Work out the finished part from the listing and answer in its coordinate system (mm). A direction names the side the tool comes from. Coordinates: 2 decimals unless noted, no trailing zeros. Order: outer loops, then holes, each group sorted by start corner. A loop starts at its lowest first (then second) coordinate and runs counter-clockwise, first axis right, second up. Notation, with made-up numbers: (36.25, 0) - (77.25, 0) arc R30 ccw to (77.25, 32) - close; hole circle Ø11 at (40.25, -6.75). An arc over 180 degrees is marked (long way). Use CSV: the item, a comma, the result in double quotes. Start each with the question number.
Autodesk Inventor part; units mm, degrees
ref_plane "YZ Plane" through (0, 0, 0) normal (1, 0, 0) x (0, 1, 0)
ref_plane "XZ Plane" through (0, 0, 0) normal (0, 1, 0) x (-1, 0, 0)
ref_plane "XY Plane" through (0, 0, 0) normal (0, 0, 1) x (1, 0, 0)
sketch "Sketch1" plane through (0, 0, 0) normal (0, 0, 1) x (1, 0, 0)
  line L0 (-105.7, 0) -> (105.7, 0) construction
  line L1 (0, -31.15) -> (0, 31.15) construction
  line L2 (-75.5, 22.25) -> (75.5, 22.25)
  line L3 (75.5, 22.25) -> (75.5, -22.25)
  line L4 (75.5, -22.25) -> (-75.5, -22.25)
  line L5 (-75.5, -22.25) -> (-75.5, 22.25)
  line L6 (-49.21, 1.55) -> (-49.21, -1.55) construction
  line L7 (-56.21, 1.55) -> (-56.21, -1.55)
  line L8 (-42.21, -1.55) -> (-42.21, 1.55)
  arc A0 (-42.21, 1.55) -> (-56.21, 1.55) centre (-49.21, 1.55) ccw
  arc A1 (-56.21, -1.55) -> (-42.21, -1.55) centre (-49.21, -1.55) ccw
  line L9 (49.21, 1.55) -> (49.21, -1.55) construction
  line L10 (56.21, 1.55) -> (56.21, -1.55)
  line L11 (42.21, -1.55) -> (42.21, 1.55)
  arc A2 (56.21, 1.55) -> (42.21, 1.55) centre (49.21, 1.55) ccw
  arc A3 (42.21, -1.55) -> (56.21, -1.55) centre (49.21, -1.55) ccw
  line L12 (-49.21, 1.55) -> (-49.21, -1.55) construction
  line L13 (-59.71, 1.55) -> (-59.71, -1.55)
  line L14 (-38.71, -1.55) -> (-38.71, 1.55)
  arc A4 (-38.71, 1.55) -> (-59.71, 1.55) centre (-49.21, 1.55) ccw
  arc A5 (-59.71, -1.55) -> (-38.71, -1.55) centre (-49.21, -1.55) ccw
  line L15 (59.71, 1.55) -> (59.71, -1.55)
  line L16 (38.71, -1.55) -> (38.71, 1.55)
  arc A6 (59.71, 1.55) -> (38.71, 1.55) centre (49.21, 1.55) ccw
  arc A7 (38.71, -1.55) -> (59.71, -1.55) centre (49.21, -1.55) ccw
  point P0 (0, 0)
  point P1 (-49.21, 0)
  point P2 (49.21, 0)
  point P3 (-49.21, 0)
  dimension "d0" = 44.5
  dimension "d1" = 151
  dimension "d26" = 14
  dimension "d27" = 20.7
  dimension "d28" = 98.42
  dimension "d29" = 21
  dimension "d30" = 1.55
extrude "Extrusion1" add sketch "Sketch1" against normal blind 22 contours L2 L3 L4 L5 | A0 L8 A1 L7 | L10 A3 L11 A2 | A4 L14 A5 L13 | L15 A7 L16 A6
extrude "Extrusion2" cut sketch "Sketch1" against normal through all contours A0 L8 A1 L7 | L10 A3 L11 A2
extrude "Extrusion3" cut sketch "Sketch1" against normal blind 16.78 contours L10 A3 L11 A2 | A4 L14 A5 L13 | L15 A7 L16 A6
chamfer "Chamfer3" distance 1 angle 45 4 edges at (0, 22.25, -22) (-75.5, 0, -22) (0, -22.25, -22) (75.5, 0, -22)
chamfer "Chamfer4" distance 1.5 angle 45 8 edges at (-49.21, 12.05, 0) (-38.71, 0, 0) (-49.21, -12.05, 0) (-59.71, 0, 0) (49.21, 12.05, 0) (59.71, 0, 0) (49.21, -12.05, 0) (38.71, 0, 0)
chamfer "Chamfer5" distance 0.5 angle 45 8 edges at (-49.21, 8.55, -22) (-56.21, 0, -22) (-49.21, -8.55, -22) (-42.21, 0, -22) (49.21, -8.55, -22) (56.21, 0, -22) (49.21, 8.55, -22) (42.21, 0, -22)
sketch "Sketch2" plane through (-75.5, 22.25, 0) normal (0, 1, 0) x (1, 0, 0)
  line L0 (0, 21) -> (151, 21) construction
  line L1 (0, 0) -> (0, 21) construction
  line L2 (151, 0) -> (0, 0)
  line L3 (151, 0) -> (151, 21) construction
  line L4 (75.5, 42.335) -> (75.5, -100.0102) construction
  circle A0 centre (75.5, -32.1751) radius 47.5 construction
  line L5 (150, 22) -> (1, 22)
  line L6 (62.5, 22) -> (40.5, 0)
  line L7 (88.5, 22) -> (110.5, 0)
  line L8 (14.29, 0) -> (38.29, 0)
  line L9 (33, 0) -> (55, 22)
  line L10 (118, 0) -> (96, 22)
  circle A1 centre (75.5, -28.2107) radius 50 construction
  line L11 (60.5, 20) -> (90.5, 20)
  dimension "d54" = 95
  dimension "d57" = 45
  dimension "d59" = 70
  dimension "d60" = 45
  dimension "d61" = 85
  dimension "d62" = 100
  dimension "d68" = 2
extrude "Extrusion6" cut sketch "Sketch2" against normal blind 35 contours L2 L6 L11 L7
extrude "Extrusion7" cut sketch "Sketch2" against normal blind 6 contours L2 L7 L5 L10 | L2 L9 L5 L6 | L11 L6 L5 L7
fillet "Fillet1" radius 10 2 edges at (-15, 1.75, -20) (15, 1.75, -20)
equation "\"d0\" = jawH"
equation "\"d1\" = jawW"
equation "\"d4\" = jawT"
equation "\"jawH\" = 44.5"
equation "\"jawW\" = 151"
equation "\"jawT\" = 22"
properties part number "JawDualSided" material "Aluminum 6061"
1) Flat-ended cylindrical pins translate along their axes: P1, Ø17, axis at x = -51, y = -5, coming from the +Z side; P2, Ø17.5, axis at x = -5.5, y = -0.5, coming from the +Z side; P3, Ø17, axis at x = 48, y = -1.5, coming from the +Z side; P4, Ø8, axis at x = 22.5, y = 6.5, coming from the +Z side. Find the tip coordinate at first contact, or state that the pin passes through.
2) Straight lines are drawn through the part: line 1 (X direction, y = 6.5, z = -9.5); line 2 (X direction, y = 4, z = -6); line 3 (Y direction, x = 50, z = -1.5). For each, find the intervals that lie inside material, in ascending order. Write a range as [from, to].
3) For faces 1 (the face through (-31.7, 19.3, -10.8)), 2 (the face through (42.21, 0, -19)), 3 (the face through (-56.4, 0.2, -16.78)), determine the directions among +Z, -Z, +X, -X, +Y, -Y from which every point of the face is accessible in a straight line to the end or side of a thin tool.
4) The part is cut by section A-A on z = -14.5. Determine the outline of the cut face in (x, y).
5) The part is cut by section B-B on x = 49.21. Determine the outline of the cut face in (y, z).
6) The part is cut by section D-D on z = -3.5. Determine the outline of the cut face in (x, y).
7) The part is cut by section C-C on x = -30. Determine the outline of the cut face in (y, z).
8) For a pull along Y with two mould halves and no side action, classify faces 4 (the face through (42, 0, -16.78)), 5 (the face through (-55, 22.25, -10)), 6 (the face through (-75.5, 0, -10)) as +Y half, -Y half, draft (parallel to the pull), parting line (faces both ways), or undercut.
Answer key:
1,P1,"z = 0"
1,P2,"z = -19.41"
1,P3,"z = -16.78"
1,P4,"z = -8.5"
2,line 1,"[-75.5, -58.47], [-39.95, -25.5], [25.5, 39.95], [58.47, 75.5]"
2,line 2,"[-75.5, -59.42], [-39, -29], [29, 39], [59.42, 75.5]"
2,line 3,"[-22.25, -12.02], [12.02, 22.25]"
3,face 1,"+Z, +Y"
3,face 2,"+Z, -Z"
3,face 3,"+Z"
4,outline,"(-75.5, -22.25) - (75.5, -22.25) - (75.5, 22.25) - (28, 22.25) - (28, 16.25) - (20.5, 16.25) - (20.5, -12.75) - (-20.5, -12.75) - (-20.5, 16.25) - (-28, 16.25) - (-28, 22.25) - (-75.5, 22.25) - close; hole (-59.71, -1.55) arc R10.5 ccw to (-38.71, -1.55) - (-38.71, 1.55) arc R10.5 ccw to (-59.71, 1.55) - close; hole (38.71, -1.55) arc R10.5 ccw to (59.71, -1.55) - (59.71, 1.55) arc R10.5 ccw to (38.71, 1.55) - close"
5,outline,"(-22.25, -21) - (-21.25, -22) - (-9.05, -22) - (-8.55, -21.5) - (-8.55, -16.78) - (-12.05, -16.78) - (-12.05, -1.5) - (-13.55, 0) - (-22.25, 0) - close; (8.55, -21.5) - (9.05, -22) - (21.25, -22) - (22.25, -21) - (22.25, 0) - (13.55, 0) - (12.05, -1.5) - (12.05, -16.78) - (8.55, -16.78) - close"
6,outline,"(-75.5, -22.25) - (75.5, -22.25) - (75.5, 22.25) - (39, 22.25) - (39, 16.25) - (31.5, 16.25) - (31.5, -12.75) - (-31.5, -12.75) - (-31.5, 16.25) - (-39, 16.25) - (-39, 22.25) - (-75.5, 22.25) - close; hole (-59.71, -1.55) arc R10.5 ccw to (-38.71, -1.55) - (-38.71, 1.55) arc R10.5 ccw to (-59.71, 1.55) - close; hole (38.71, -1.55) arc R10.5 ccw to (59.71, -1.55) - (59.71, 1.55) arc R10.5 ccw to (38.71, 1.55) - close"
7,outline,"(-22.25, -21) - (-21.25, -22) - (21.25, -22) - (22.25, -21) - (22.25, -12.5) - (16.25, -12.5) - (16.25, -5) - (-12.75, -5) - (-12.75, 0) - (-22.25, 0) - close"
8,face 4,"undercut"
8,face 5,"+Y half"
8,face 6,"draft"
